Build history of the part. All positions in model axes, mm. A direction names the side the tool comes from. Give positions to 0.01 mm unless a question says otherwise; leave off trailing zeros. Order: outer loops, then holes, each group sorted by start corner. A loop starts at its lowest first (then second) coordinate and runs counter-clockwise, first axis right, second up. Notation, with made-up numbers: (-11.5, 35) -> (27.5, 35) arc R30 cw to (27.5, 61) -> close; hole circle Ø8 at (89, 52). An arc over 180 degrees is marked (long way). One line per question, with ' | ' between items. Start each with the question number.
(1) Pin check, flat tips, straight feed: pin 1 Ø5 at (x, z) = (6.5, -7) entering from +Y; pin 2 Ø1.5 at (x, z) = (6.5, -16.5) entering from -Y; pin 3 Ø12 at (x, z) = (8.5, -9) entering from +Y. Stop position of each tip, or through.
(2) Pull direction Z, two halves, no side cores. Call faces 3 (the face through (8.105, 7.201, -17.457)), 4 (the face through (8, 2.929, -8)), 5 (the face through (8, 5, 6.814)), 6 (the face through (-5, 10, -8)): +Z half, -Z half, draft (parallel to the pull), parting line (faces both ways), or undercut.
(3) Cut at A-A (y = 7). Give the cut face in (x, z), then the cut area to 3 significant figures.
(4) Cut at C-C (z = -18.5). Give the cut face in (x, y).
(5) Drill centre lines: L1, parallel to X at y = 6, z = -8; L2, parallel to X at y = 9.5, z = -17.75; L3, parallel to Z at x = 6.75, y = 5.75. Where is each one in solid material? Low to high. Write a range as from..to.
(6) Which spindle directions (+Z, -Z, +X, -X, +Y, -Y) get a long thin tool onto all of the face, cutting with end or side? Do faces 1 (the face through (7.767, 7.201, 1.086)), 2 (the face through (22.936, 5, -8)). Say none if no direction does.
Autodesk Inventor part; units mm, degrees
ref_plane "YZ Plane" through (0, 0, 0) normal (1, 0, 0) x (0, 1, 0)
ref_plane "XZ Plane" through (0, 0, 0) normal (0, 1, 0) x (-1, 0, 0)
ref_plane "XY Plane" through (0, 0, 0) normal (0, 0, 1) x (1, 0, 0)
sketch "Sketch1" plane through (0, 0, 0) normal (0, 1, 0) x (-1, 0, 0)
  line L0 (7.064, 6.8143) -> (-22.936, 6.8143)
  line L1 (-22.936, 6.8143) -> (-22.936, -23.1857)
  line L2 (-22.936, -23.1857) -> (7.064, -23.1857)
  line L3 (7.064, -23.1857) -> (7.064, 6.8143)
  point P0 (0, 0)
  dimension "d0" = 30
  dimension "d1" = 30
extrude "Extrusion1" add sketch "Sketch1" along normal blind 10
sketch "Sketch2" plane through (0, 10, 0) normal (0, 1, 0) x (1, 0, 0)
  point P0 (0, 0)
sketch "Sketch3" plane through (0, 10, 0) normal (0, 1, 0) x (1, 0, 0)
  line L0 (2.936, 13.1857) -> (12.936, 13.1857)
  line L1 (12.936, 13.1857) -> (12.936, 3.1857)
  line L2 (12.936, 3.1857) -> (2.936, 3.1857)
  line L3 (2.936, 3.1857) -> (2.936, 13.1857)
  line L4 (22.936, -6.8143) -> (22.936, 23.1857)
  line L5 (-7.064, -6.8143) -> (22.936, -6.8143)
  point P0 (0, 0)
  dimension "d4" = 10
  dimension "d5" = 10
  dimension "d6" = 10
  dimension "d7" = 10
extrude "Extrusion2" cut sketch "Sketch3" against normal blind 7.0711
chamfer "Chamfer1" distance 7.0711 distance2 7.0711 1 edges at (7.936, 10, -13.1857) measured on face at (6.2693, 10, -19.8524)
chamfer "Chamfer2" distance 7.0711 distance2 7.0711 1 edges at (2.936, 10, -8.1857) measured on face at (-3.7307, 10, -9.8524)
chamfer "Chamfer3" distance 7.0711 distance2 7.0711 1 edges at (7.936, 10, -3.1857) measured on face at (9.6026, 10, 3.481)
chamfer "Chamfer4" distance 7.0711 distance2 7.0711 1 edges at (12.936, 10, -8.1857) measured on face at (19.6026, 10, -9.8524)
sketch "Sketch4" plane through (-4.1351, 10, -20.2568) normal (0.7071, 0.7071, 0) x (-0.7071, 0.7071, 0)
  circle A0 centre (-5, 12.0711) radius 5
  line L0 (0, 0) -> (0, 24.1421)
  point P0 (-9.995, 20.2568)
  dimension "d22" = 10
  dimension "d23" = 0
  dimension "d24" = 24.1421
  dimension "d25" = 12.0711
equation "\"d7\" = d6"
equation "\"d25\" = 0.5 * d24"
Result set:
1) pin 1: stops at y = 2.93 | pin 2: stops at y = 0 | pin 3: stops at y = 4.74
2) face 3: undercut | face 4: undercut | face 5: +Z half | face 6: draft
3) outline: (-7.06, -23.19) -> (22.94, -23.19) -> (22.94, 6.81) -> (-7.06, 6.81) -> close; hole (-1.13, -17.26) -> (17.01, -17.26) -> (17.01, 0.88) -> (-1.13, 0.88) -> close | area: 571 mm2
4) outline: (-7.06, 0) -> (22.94, 0) -> (22.94, 10) -> (20.01, 10) -> (18.25, 8.24) -> (-2.38, 8.24) -> (-4.13, 10) -> (-7.06, 10) -> close
5) L1: x = -7.06..-0.13, 16.01..22.94 | L2: x = -7.06..-3.63, 19.51..22.94 | L3: z = -23.19..-16.01, -0.37..6.81
6) face 1: +Y | face 2: +Z, -Z, +X, +Y, -Y
